```python
from build123d import *

# Parameters (mm, degrees)
BOSS_EXTRU_1_DEPTH       = 8
ESQUISSE4_W              = 82
ESQUISSE4_H              = 12
ENL_V_MAT_EXTRU_3_DEPTH  = 9
BOSS_EXTRU_2_REACH       = 18
ESQUISSE6_W              = 4.318
ESQUISSE6_H              = 8
ESQUISSE7_R              = 1.3
ENL_V_MAT_EXTRU_5_DEPTH  = 10
ESQUISSE8_W              = 5.09860661
ESQUISSE8_H              = 12
ESQUISSE8_W_2            = 4.318
ENL_V_MAT_EXTRU_6_DEPTH  = 3
ESQUISSE13_R             = 4
ENL_V_MAT_EXTRU_9_DEPTH  = 4.3
ENL_V_MAT_EXTRU_10_DEPTH = 4.3
ESQUISSE15_R             = 2.5
ENL_V_MAT_EXTRU_11_DEPTH = 3.4
ENL_V_MAT_EXTRU_12_REACH = 6.6
ESQUISSE16_R             = 1.25
ESQUISSE17_W             = 24.484825334
ESQUISSE17_H             = 8
ENL_V_MAT_EXTRU_13_DEPTH = 4.3
ESQUISSE18_W             = 4.318
ESQUISSE18_H             = 12
ENL_V_MAT_EXTRU_14_DEPTH = 3


with BuildPart() as part:
    # Esquisse1 → Boss.-Extru.1 (new body)
    with BuildSketch(Plane.XY):
        with BuildLine():
            Line((0, 0), (100, 0))
            ThreePointArc((100, 0), (110, 10), (100, 20))
            Line((100, 20), (0, 20))
            ThreePointArc((0, 20), (-10, 10), (0, 0))
        make_face()
    extrude(amount=BOSS_EXTRU_1_DEPTH)

    # Esquisse4 → Enlèv. mat.-Extru.3 (cut, through all)
    with BuildSketch(Plane.XY.offset(8)):
        with Locations((49, 10)):
            Rectangle(ESQUISSE4_W, ESQUISSE4_H)
    extrude(amount=-ENL_V_MAT_EXTRU_3_DEPTH, mode=Mode.SUBTRACT)

    # Esquisse6 → Boss.-Extru.2 (add, up to next)
    with BuildSketch(Plane(origin=(0, 4, 0), x_dir=(1, 0, 0), z_dir=(0, 1, 0)), mode=Mode.PRIVATE) as boss_extru_2_sk1:
        with Locations((63.356174666, -4)):
            Rectangle(ESQUISSE6_W, ESQUISSE6_H)
    boss_extru_2_tool1 = extrude(boss_extru_2_sk1.sketch, amount=BOSS_EXTRU_2_REACH, mode=Mode.PRIVATE) - part.part
    add(boss_extru_2_tool1.solids().sort_by_distance((63.356175, 4, 4))[0])

    # Esquisse7 → Enlèv. mat.-Extru.5 (cut)
    with BuildSketch(Plane(origin=(0, 0, 0), x_dir=(-1, 0, 0), z_dir=(0, 0, -1))):
        with Locations((-91.542174666, 13.344)):
            Circle(ESQUISSE7_R)
        with Locations((-91.542174666, 6.74)):
            Circle(ESQUISSE7_R)
        with Locations((-63.973, 6.74)):
            Circle(ESQUISSE7_R)
        with Locations((-63.973, 13.344)):
            Circle(ESQUISSE7_R)
    extrude(amount=-ENL_V_MAT_EXTRU_5_DEPTH, mode=Mode.SUBTRACT)

    # Esquisse8 → Enlèv. mat.-Extru.6 (cut)
    with BuildSketch(Plane.XY.offset(8)):
        with Locations((92.549303305, 10)):
            Rectangle(ESQUISSE8_W, ESQUISSE8_H)
        with Locations((63.356174666, 10)):
            Rectangle(ESQUISSE8_W_2, ESQUISSE8_H)
    extrude(amount=-ENL_V_MAT_EXTRU_6_DEPTH, mode=Mode.SUBTRACT)

    # Esquisse13 → Enlèv. mat.-Extru.9 (cut)
    with BuildSketch(Plane.XY.offset(8)):
        with Locations((0, 10)):
            Circle(ESQUISSE13_R)
    extrude(amount=-ENL_V_MAT_EXTRU_9_DEPTH, mode=Mode.SUBTRACT)

    # Esquisse14 → Enlèv. mat.-Extru.10 (cut)
    with BuildSketch(Plane.XY.offset(8)):
        Polygon((2.655377087, 4.544050257), (2.655377087, -2.008601379), (-2.844622913, -1.912365766), (-2.844622913, 4.640285869), (-5.455949743, 7.344622913), (-12.008601379, 7.344622913), (-11.912365766, 12.844622913), (-5.359714131, 12.844622913), (-2.655377087, 15.455949743), (-2.655377087, 22.008601379), (2.844622913, 21.912365766), (2.844622913, 15.359714131), (5.455949743, 12.655377087), (12.008601379, 12.655377087), (11.912365766, 7.155377087), (5.359714131, 7.155377087), align=None)
    extrude(amount=-ENL_V_MAT_EXTRU_10_DEPTH, mode=Mode.SUBTRACT)

    # Esquisse15 → Enlèv. mat.-Extru.11 (cut)
    with BuildSketch(Plane(origin=(0, 0, 0), x_dir=(-1, 0, 0), z_dir=(0, 0, -1))):
        with Locations((0, 10)):
            Circle(ESQUISSE15_R)
    extrude(amount=-ENL_V_MAT_EXTRU_11_DEPTH, mode=Mode.SUBTRACT)

    # Esquisse16 → Enlèv. mat.-Extru.12 (cut, up to next)
    with BuildSketch(Plane(origin=(0, 0, 3.4), x_dir=(-1, 0, 0), z_dir=(0, 0, -1)), mode=Mode.PRIVATE) as enl_v_mat_extru_12_sk1:
        with Locations((0, 10)):
            Circle(ESQUISSE16_R)
    enl_v_mat_extru_12_tool1 = extrude(enl_v_mat_extru_12_sk1.sketch, amount=-ENL_V_MAT_EXTRU_12_REACH, mode=Mode.PRIVATE) & part.part
    add(enl_v_mat_extru_12_tool1.solids().sort_by_distance((0, 10, 3.4))[0], mode=Mode.SUBTRACT)

    # Esquisse17 → Enlèv. mat.-Extru.13 (cut)
    with BuildSketch(Plane(origin=(0, 20, 0), x_dir=(1, 0, 0), z_dir=(0, 1, 0))):
        with Locations((77.757587333, -4)):
            Rectangle(ESQUISSE17_W, ESQUISSE17_H)
    extrude(amount=-ENL_V_MAT_EXTRU_13_DEPTH, mode=Mode.SUBTRACT)

    # Esquisse18 → Enlèv. mat.-Extru.14 (cut)
    with BuildSketch(Plane(origin=(0, 0, 0), x_dir=(-1, 0, 0), z_dir=(0, 0, -1))):
        with Locations((-63.356174666, 10)):
            Rectangle(ESQUISSE18_W, ESQUISSE18_H)
        with Locations((-92.159, 10)):
            Rectangle(ESQUISSE18_W, ESQUISSE18_H)
    extrude(amount=-ENL_V_MAT_EXTRU_14_DEPTH, mode=Mode.SUBTRACT)


solid = part.part
```
Work out the finished part from the listing and answer in its coordinate system (mm). A direction names the side the tool comes from. Round coordinates to 2 decimals unless told otherwise and drop trailing zeros. Order: outer loops, then holes, each group sorted by start corner. A loop starts at its lowest first (then second) coordinate and runs counter-clockwise, first axis right, second up.
Q1. Find the intervals of material crossed by line 1 along Y through (x, z) = (30, 6); line 2 along Y through (x, z) = (0, 1.55); line 3 along X through (y, z) = (12, 2.5), in increasing order.
Solution:
line 1: y = 0 to 4, 16 to 20
line 2: y = 0 to 7.5, 12.5 to 20
line 3: x = -9.8 to -1.5, 1.5 to 8, 94.32 to 109.8
Q2. A tool of negligible diameter and unlimited length cuts with its end or side. For faces 1 (the flat face through (8, 10, 3)), 2 (the flat face through (4.13, 14.03, 5.88)), 3 (the cylindrical face through (0.54, 7.56, 1.68)), from which of +Z, -Z, +X, -X, +Y, -Y can it reach the whole face along a straight path? Write none if from no direction.
Solution:
face 1: +Z, -Z
face 2: +Z
face 3: -Z
Q3. A cutting plane is placed at B-B, the plane x = 15.5. Determine the outline of the cut face in (y, z), then the cut area to 3 significant figures.
Solution:
outline: (0, 0) - (4, 0) - (4, 8) - (0, 8) - close; (16, 0) - (20, 0) - (20, 8) - (16, 8) - close
area: 64.0 mm2
Q4. The mould has two halves that part along X. Classify faces 4 (the flat face through (-4.03, 14.13, 5.88)), 5 (the cylindrical face through (-10, 10, 3)), 6 (the cylindrical face through (110, 10, 4)): pulls with the +X half, pulls with the -X half, needs draft (parallel to the pull), parting line crosses it, or undercut.
Solution:
face 4: undercut
face 5: pulls with the -X half
face 6: pulls with the +X half
Q5. Given pin 1 Ø3.5 at (y, z) = (17, 5) entering from +X; pin 2 Ø1.5 at (x, y) = (88, 5.5) entering from -Z; pin 3 Ø3 at (x, y) = (91.54, 6.74) entering from -Z; pin 4 Ø2 at (y, z) = (12, 4) entering from -X, each flat-ended and moving along its own axis, determine where each tip first touches the part or whether it passes through.
Solution:
pin 1: stops at x = 108.51
pin 2: passes through
pin 3: stops at z = 3
pin 4: stops at x = -9.95
Q6. A cutting plane is placed at A-A, the plane y = 10. Determine the outline of the cut face in (x, z), then the cut area to 3 significant figures.
Solution:
outline: (-10, 0) - (-2.5, 0) - (-2.5, 3.4) - (-1.25, 3.4) - (-1.25, 3.7) - (-10, 3.7) - close; (1.25, 3.4) - (2.5, 3.4) - (2.5, 0) - (8, 0) - (8, 3.7) - (1.25, 3.7) - close; (61.2, 3) - (65.52, 3) - (65.52, 5) - (61.2, 5) - close; (90, 3) - (94.32, 3) - (94.32, 0) - (110, 0) - (110, 8) - (95.1, 8) - (95.1, 5) - (90, 5) - close
area: 189 mm2
